Can you work these out from the model? Positions are in its coordinate system, mm. Face numbers are marked on the shaded views. A direction names the side the tool comes from. Round coordinates to 2 decimals unless told otherwise and drop trailing zeros. Write each loop counter-clockwise with the first axis right and the second up, starting at its lowest first coordinate (ties: lowest second). Pieces come first, ordered by that corner, then holes. Notation, with made-up numbers: (86.5, 89.25) -> (96.5, 89.25) arc R22 cw to (96.5, 105.25) -> close; hole circle Ø10 at (-13.5, -37.5). An arc over 180 degrees is marked (long way). Write item = value, one per line. Start each with the question number.
1) For the marked faces 4, 5, 6 and 7, which set-ups out of +Z, -Z, +X, -X, +Y, -Y let a thin tool reach every point of the face, with its end or its side?
2) Thinking about a two-plate mould opening in X: for the marked faces 1, 2 and 3, which applies, +X half, -X half, draft (parallel to the pull), parting line (faces both ways), or undercut?
3) I'm going to push flat-ended pins straight in: pin 1 (4 mm diameter, centred on y = -11.5, z = 6, fed in from +X); pin 2 (7 mm diameter, centred on y = -8.5, z = -17, fed in from -X); pin 3 (1.5 mm diameter, centred on x = -8.5, z = 6.5, fed in from -Y); pin 4 (8 mm diameter, centred on y = 16.5, z = -10, fed in from -X). Where does each tip first touch, or does it pass through?
4) Imagine slicing it at C-C, the plane y = -8.5. Please give me the cut outline in (x, z), then the cut area to 3 significant figures.
5) If I drill on line 1 (Z direction, x = -44, y = -8); line 2 (X direction, y = 23, z = 4); line 3 (X direction, y = -13, z = 17), over which ranges is the centre line in solid material (lowest first)?
6) Imagine slicing it at A-A, the plane y = 0. Please give me the cut outline in (x, z).
7) Imagine slicing it at D-D, the plane z = -22. Please give me the cut outline in (x, y), then the cut area to 3 significant figures.
8) Imagine slicing it at B-B, the plane z = 17. Please give me the cut outline in (x, y), then the cut area to 3 significant figures.
from build123d import *
from OCP.BRepAlgoAPI import BRepAlgoAPI_Cut
from OCP.TopTools import TopTools_ListOfShape
from build123d.topology import SkipClean

# Parameters (mm, degrees)
BOSS_EXTRUDE1_DEPTH      = 26
BOSS_EXTRUDE1_DEPTH_BACK = 26
SKETCH1_W                = 6
SKETCH1_H                = 22
SKETCH2_W                = 17
SKETCH2_H                = 45.409673579
CUT_EXTRUDE1_DEPTH       = 60
SKETCH3_R                = 4
CUT_EXTRUDE2_DEPTH       = 12.000001
SKETCH4_W                = 12
SKETCH4_H                = 22
CUT_EXTRUDE4_DEPTH       = 18
CUT_EXTRUDE5_START       = -5
CUT_EXTRUDE5_DEPTH       = 5
CUT_EXTRUDE6_DEPTH       = 5
SKETCH8_R                = 2.5
CUT_EXTRUDE7_DEPTH       = 3
SKETCH9_W                = 18.588465887
SKETCH9_H                = 5
CUT_EXTRUDE8_DEPTH       = 22
FILLET2_RADIUS           = 9
FILLET2_LENGTH           = 3.00000065
FILLET3_RADIUS           = 9
FILLET3_LENGTH           = 3
CUT_EXTRUDE9_START       = -5
CUT_EXTRUDE9_DEPTH       = 5
BOSS_EXTRUDE2_START      = -5
SKETCH11_R               = 17.5
SKETCH11_R_2             = 12.5
BOSS_EXTRUDE2_DEPTH      = 5
CUT_EXTRUDE10_DEPTH      = 5
SKETCH13_R               = 17.5
SKETCH13_R_2             = 12.5
BOSS_EXTRUDE3_DEPTH      = 5
CUT_EXTRUDE11_START      = -18
SKETCH14_W               = 3
SKETCH14_H               = 6.500000134
CUT_EXTRUDE11_DEPTH      = 18
SKETCH15_R               = 3.2
CUT_EXTRUDE12_DEPTH      = 3.000001


with BuildPart() as part:
    # Sketch1 → Boss-Extrude1 (new, two sides: drawn at the far end of the back side and taken through both)
    with BuildSketch(Plane.XY.offset(-BOSS_EXTRUDE1_DEPTH_BACK)):
        with Locations((-44.500000239, -6.499999432)):
            Rectangle(SKETCH1_W, SKETCH1_H)
        with BuildLine():
            ThreePointArc((-2.39e-07, -17.5), (-16.878212154, -4.623413726), (-8.918281091, 15.057033652))
            Line((-8.918281091, 15.057033652), (-47.500000239, 4.500000568))
            Line((-47.500000239, 4.500000568), (-41.500000239, 4.500000568))
            Line((-41.500000239, 4.500000568), (-41.500000239, -17.499999432))
            Line((-41.500000239, -17.499999432), (-2.39e-07, -17.5))
        make_face()
        with BuildLine():
            Line((-4.500000094, 27.909673713), (-4.500000094, 16.9115345))
            ThreePointArc((-4.500000094, 16.9115345), (-2.39e-07, -17.5), (4.500000556, 16.911534377))
            Line((4.500000556, 16.911534377), (4.500000556, 27.909673579))
            Line((4.500000556, 27.909673579), (1.500000556, 27.909673579))
            Line((1.500000556, 27.909673579), (1.500000556, 12.409673579))
            ThreePointArc((1.500000556, 12.409673579), (-5.6e-07, -12.5), (-1.499999444, 12.409673713))
            Line((-1.499999444, 12.409673713), (-1.499999444, 27.909673713))
            Line((-1.499999444, 27.909673713), (-4.500000094, 27.909673713))
        make_face()
    extrude(amount=BOSS_EXTRUDE1_DEPTH + BOSS_EXTRUDE1_DEPTH_BACK)

    # Sketch2 → Cut-Extrude1 (cut)
    with BuildSketch(Plane(origin=(24.500000556, 0, 0), x_dir=(0, 0, -1), z_dir=(1, 0, 0))):
        with Locations((-17.5, 5.20483679)):
            Rectangle(SKETCH2_W, SKETCH2_H)
        with Locations((17.5, 5.20483679)):
            Rectangle(SKETCH2_W, SKETCH2_H)
    extrude(amount=-CUT_EXTRUDE1_DEPTH, mode=Mode.SUBTRACT)

    # Sketch3 → Cut-Extrude2 (cut)
    with BuildSketch(Plane.ZY.offset(47.500000239)):
        with Locations((-17, -8.499999432)):
            Circle(SKETCH3_R)
        with Locations((17, -8.499999432)):
            Circle(SKETCH3_R)
    extrude(amount=-CUT_EXTRUDE2_DEPTH, mode=Mode.SUBTRACT)


with BuildPart() as cut_extrude4_tool:
    # Sketch4 → Cut-Extrude4 (new body)
    with BuildSketch(Plane(origin=(3.08e-07, 22.5, 0), x_dir=(-0.9999999999999999, 1.3684242577770874e-08, 0), z_dir=(-1.3684242577770874e-08, -0.9999999999999999, 0))):
        with Locations((41.500000301, 15)):
            Rectangle(SKETCH4_W, SKETCH4_H)
        with Locations((41.500000301, -15)):
            Rectangle(SKETCH4_W, SKETCH4_H)
    extrude(amount=CUT_EXTRUDE4_DEPTH)


with BuildPart() as part_1:
    add(part.part)

    # Cut-Extrude4: cut by cut_extrude4_tool, with a tolerance
    cut_extrude4_stock = TopTools_ListOfShape()
    cut_extrude4_stock.Append(part_1.part.wrapped)
    cut_extrude4_tools = TopTools_ListOfShape()
    cut_extrude4_tools.Append(cut_extrude4_tool.part.wrapped)
    cut_extrude4_cut = BRepAlgoAPI_Cut()
    cut_extrude4_cut.SetArguments(cut_extrude4_stock)
    cut_extrude4_cut.SetTools(cut_extrude4_tools)
    cut_extrude4_cut.SetFuzzyValue(0.00001)
    cut_extrude4_cut.Build()
    add(Compound.cast(cut_extrude4_cut.Shape()).solids(), mode=Mode.REPLACE)

    # Sketch5 → Cut-Extrude5 (cut)
    with BuildSketch(Plane.XY.offset(9).offset(CUT_EXTRUDE5_START)):
        with BuildLine():
            Line((-47.500000239, 4.50000065), (-16.911534352, 4.50000065))
            ThreePointArc((-16.911534352, 4.50000065), (-13.951973972, 10.563731456), (-8.918281071, 15.057033663))
            Line((-8.918281071, 15.057033663), (-47.500000239, 4.50000065))
        make_face()
    extrude(amount=CUT_EXTRUDE5_DEPTH, mode=Mode.SUBTRACT)

    # Sketch7 → Cut-Extrude6 (cut)
    with BuildSketch(Plane(origin=(0, 0, -9), x_dir=(-1, 0, 0), z_dir=(0, 0, -1))):
        with BuildLine():
            Line((47.500000239, 4.50000065), (16.911534352, 4.50000065))
            ThreePointArc((16.911534352, 4.50000065), (13.951973972, 10.563731456), (8.918281071, 15.057033663))
            Line((8.918281071, 15.057033663), (47.500000239, 4.50000065))
        make_face()
    extrude(amount=-CUT_EXTRUDE6_DEPTH, mode=Mode.SUBTRACT)

    # Sketch8 → Cut-Extrude7 (cut)
    with BuildSketch(Plane(origin=(4.500000556, 0, 0), x_dir=(0, 0, -1), z_dir=(1, 0, 0))):
        with Locations(Location((0, 22.410603978, 0), (0, 0, 90))):
            Circle(SKETCH8_R)
    extrude(amount=-CUT_EXTRUDE7_DEPTH, mode=Mode.SUBTRACT)


with BuildPart() as cut_extrude8_tool:
    # Sketch9 → Cut-Extrude8 (new body)
    with BuildSketch(Plane(origin=(6.2e-08, 4.5, 0), x_dir=(1.0, -1.3684242685755665e-08, 0), z_dir=(1.3684242685755665e-08, 1.0, 0))):
        with Locations((-26.205767358, 6.5)):
            Rectangle(SKETCH9_W, SKETCH9_H)
        with Locations((-26.205767358, -6.5)):
            Rectangle(SKETCH9_W, SKETCH9_H)
    extrude(amount=-CUT_EXTRUDE8_DEPTH)


with BuildPart() as part_2:
    add(part_1.part)

    # Cut-Extrude8: cut by cut_extrude8_tool, with a tolerance
    cut_extrude8_stock = TopTools_ListOfShape()
    cut_extrude8_stock.Append(part_2.part.wrapped)
    cut_extrude8_tools = TopTools_ListOfShape()
    cut_extrude8_tools.Append(cut_extrude8_tool.part.wrapped)
    cut_extrude8_cut = BRepAlgoAPI_Cut()
    cut_extrude8_cut.SetArguments(cut_extrude8_stock)
    cut_extrude8_cut.SetTools(cut_extrude8_tools)
    cut_extrude8_cut.SetFuzzyValue(0.00001)
    cut_extrude8_cut.Build()
    add(Compound.cast(cut_extrude8_cut.Shape()).solids(), mode=Mode.REPLACE)

    # Fillet2: full round fillet: the end face becomes a half cylinder, R = half its width
    fillet2_face = Plane((-2.999999769, 27.909673579, 0), x_dir=(-1, 0, 0), z_dir=(0, 1, 0))  # on the end face: x along it, z out of the body
    fillet2_slab = fillet2_face.offset(-FILLET2_RADIUS / 2) * Box(FILLET2_LENGTH, 2 * FILLET2_RADIUS, FILLET2_RADIUS, mode=Mode.PRIVATE)  # the body's end, R deep
    fillet2_round = Plane((-2.999999769, 18.909673579, 0), x_dir=(0, 1, 0), z_dir=(-1, 0, 0)) * Cylinder(FILLET2_RADIUS, FILLET2_LENGTH, mode=Mode.PRIVATE)  # its axis R under the face
    add(fillet2_slab - fillet2_round, mode=Mode.SUBTRACT)

    # Fillet3: full round fillet: the end face becomes a half cylinder, R = half its width
    fillet3_face = Plane((3.000000556, 27.909673579, 0), x_dir=(-1, 0, 0), z_dir=(0, 1, 0))  # on the end face: x along it, z out of the body
    fillet3_slab = fillet3_face.offset(-FILLET3_RADIUS / 2) * Box(FILLET3_LENGTH, 2 * FILLET3_RADIUS, FILLET3_RADIUS, mode=Mode.PRIVATE)  # the body's end, R deep
    fillet3_round = Plane((3.000000556, 18.909673579, 0), x_dir=(0, 1, 0), z_dir=(-1, 0, 0)) * Cylinder(FILLET3_RADIUS, FILLET3_LENGTH, mode=Mode.PRIVATE)  # its axis R under the face
    add(fillet3_slab - fillet3_round, mode=Mode.SUBTRACT)

    # Sketch10 → Cut-Extrude9 (cut)
    with BuildSketch(Plane.XY.offset(9).offset(CUT_EXTRUDE9_START)):
        with BuildLine():
            Line((0, -17.5), (-16.911534475, -17.5))
            Line((-16.911534475, -17.5), (-16.911534475, -4.500000187))
            ThreePointArc((-16.911534475, -4.500000187), (-10.665364427, -13.874436985), (0, -17.5))
        make_face()
    extrude(amount=CUT_EXTRUDE9_DEPTH, mode=Mode.SUBTRACT)

    # Sketch11 → Boss-Extrude2 (add)
    with BuildSketch(Plane.XY.offset(9).offset(BOSS_EXTRUDE2_START)):
        Circle(SKETCH11_R)
        with Locations(Location((0, 0, 0), (0, 0, 83.107894852))):
            Circle(SKETCH11_R_2, mode=Mode.SUBTRACT)
    extrude(amount=BOSS_EXTRUDE2_DEPTH)

    # Sketch12 → Cut-Extrude10 (cut)
    with BuildSketch(Plane(origin=(0, 0, -9), x_dir=(-1, 0, 0), z_dir=(0, 0, -1))):
        with BuildLine():
            Line((0, -17.5), (16.911534475, -17.5))
            Line((16.911534475, -17.5), (16.911534475, -4.500000187))
            ThreePointArc((16.911534475, -4.500000187), (10.665364427, -13.874436985), (0, -17.5))
        make_face()
    extrude(amount=-CUT_EXTRUDE10_DEPTH, mode=Mode.SUBTRACT)

    # Sketch13 → Boss-Extrude3 (add)
    with BuildSketch(Plane(origin=(0, 0, -9), x_dir=(-1, 0, 0), z_dir=(0, 0, -1))):
        Circle(SKETCH13_R)
        with Locations(Location((0, 0, 0), (0, 0, 180))):
            Circle(SKETCH13_R_2, mode=Mode.SUBTRACT)
    extrude(amount=-BOSS_EXTRUDE3_DEPTH)

    # Sketch14 → Cut-Extrude11 (cut)
    with SkipClean():  # the faces are left unmerged after this step: merging them gives an invalid solid
        with BuildSketch(Plane.XY.offset(9).offset(CUT_EXTRUDE11_START)):
            with Locations((5.56e-07, 15.659673646)):
                Rectangle(SKETCH14_W, SKETCH14_H)
        extrude(amount=CUT_EXTRUDE11_DEPTH, mode=Mode.SUBTRACT)

    # Sketch15 → Cut-Extrude12 (cut)
    with SkipClean():  # the faces are left unmerged after this step: merging them gives an invalid solid
        with BuildSketch(Plane.ZY.offset(4.500000094)):
            with Locations((0, 22.41060404)):
                Circle(SKETCH15_R)
        extrude(amount=-CUT_EXTRUDE12_DEPTH, mode=Mode.SUBTRACT)


solid = part_2.part
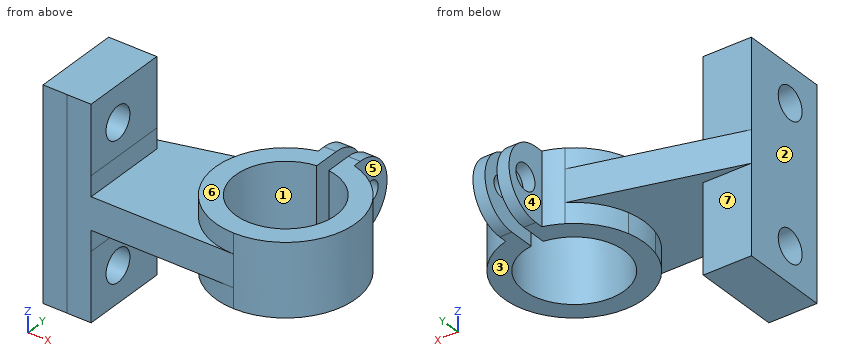
Reported:
q1.face_4 = +Z, -Z, -X, +Y
q1.face_5 = +Z, -Z, +X, +Y
q1.face_6 = +Z, +X, +Y, -Y
q1.face_7 = -Z, -X, +Y
q2.face_1 = undercut
q2.face_2 = -X half
q2.face_3 = draft
q3.pin_1 = 14.7
q3.pin_2 = through
q3.pin_3 = -15.69
q3.pin_4 = -12.12
q4.outline = (-47.5, -26) -> (-35.5, -26) -> (-35.5, -21) -> (-47.5, -21) -> close; (-47.5, -13) -> (-35.5, -13) -> (-35.5, -4) -> (-15.3, -4) -> (-15.3, -9) -> (-9.17, -9) -> (-9.17, 9) -> (-15.3, 9) -> (-15.3, 4) -> (-35.5, 4) -> (-35.5, 13) -> (-47.5, 13) -> close; (-47.5, 21) -> (-35.5, 21) -> (-35.5, 26) -> (-47.5, 26) -> close; (9.17, -9) -> (15.3, -9) -> (15.3, 9) -> (9.17, 9) -> close
q4.area = 814 mm²
q5.line_1 = -26 to -20.97, -13.03 to 13.03, 20.97 to 26
q5.line_2 = -4.5 to -1.5, 1.5 to 4.5
q5.line_3 = -47.5 to -35.5
q6.outline = (-47.5, -26) -> (-35.5, -26) -> (-35.5, -4) -> (-17.5, -4) -> (-17.5, -9) -> (-12.5, -9) -> (-12.5, 9) -> (-17.5, 9) -> (-17.5, 4) -> (-35.5, 4) -> (-35.5, 26) -> (-47.5, 26) -> close; (12.5, -9) -> (17.5, -9) -> (17.5, 9) -> (12.5, 9) -> close
q7.outline = (-47.5, -17.5) -> (-35.5, -17.5) -> (-35.5, 4.5) -> (-47.5, 4.5) -> close
q7.area = 264 mm²
q8.outline = (-47.5, -17.5) -> (-35.5, -17.5) -> (-35.5, -12.5) -> (-47.5, -12.5) -> close; (-47.5, -4.5) -> (-35.5, -4.5) -> (-35.5, 4.5) -> (-47.5, 4.5) -> close
q8.area = 168 mm²
